Autodesk Inventor part; units mm, degrees
ref_plane "YZ Plane" through (0, 0, 0) normal (1, 0, 0) x (0, 1, 0)
ref_plane "XZ Plane" through (0, 0, 0) normal (0, 1, 0) x (-1, 0, 0)
ref_plane "XY Plane" through (0, 0, 0) normal (0, 0, 1) x (1, 0, 0)
sketch "Sketch1" plane through (0, 0, -12.5) normal (0, 1, 0) x (-1, 0, 0)
  line L0 (-27.5, 12.5) -> (27.5, 12.5)
  line L1 (27.5, 12.5) -> (27.5, 37.5)
  line L2 (27.5, 37.5) -> (15.5, 37.5)
  line L3 (15.5, 37.5) -> (18.5, 31.5)
  line L4 (18.5, 31.5) -> (-18.5, 31.5)
  line L5 (-18.5, 31.5) -> (-15.5, 37.5)
  line L6 (-15.5, 37.5) -> (-27.5, 37.5)
  line L7 (-27.5, 37.5) -> (-27.5, 12.5)
  line L8 (0, 7.5) -> (0, 42.5)
  line L9 (-38.5, 12.5) -> (38.5, 12.5)
  point P0 (0, 12.5)
  point P1 (0, 12.5)
  dimension "Base_Width" = 55
  dimension "Base_Height" = 25
  dimension "Slider_Shelf" = 12
  dimension "d3" = 9
  dimension "d2" = 6
extrude "Extrusion1" add sketch "Sketch1" along normal mid plane 120
sketch "Sketch4" plane through (-18.5, 60, 19) normal (0, 0, 1) x (1, 0, 0)
  line L0 (11, -110) -> (26, -110)
  line L1 (31, -105) -> (31, -15)
  line L2 (26, -10) -> (11, -10)
  line L3 (6, -15) -> (6, -105)
  arc A0 (6, -105) -> (11, -110) centre (11, -105) ccw
  arc A1 (26, -110) -> (31, -105) centre (26, -105) ccw
  arc A2 (31, -15) -> (26, -10) centre (26, -15) ccw
  arc A3 (11, -10) -> (6, -15) centre (11, -15) ccw
  line L4 (-20, -60) -> (57, -60)
  line L5 (18.5, 24) -> (18.5, -144)
  line L6 (-9, -120) -> (-9, 0)
  line L7 (37, 0) -> (0, 0)
  dimension "StopPlate_DP" = 5
  dimension "d25" = 100
  dimension "d26" = 25
extrude "Extrusion2" cut sketch "Sketch4" against normal through all
sketch "Sketch6" plane through (0, -60, -12.5) normal (0, -1, 0) x (1, 0, 0)
  line L0 (27.5, 37.5) -> (27.5, 12.5)
  line L1 (-27.5, 12.5) -> (27.5, 12.5)
  line L2 (27.5, 12.5) -> (27.5, 57)
  line L3 (27.5, 57) -> (-27.5, 57)
  line L4 (-27.5, 57) -> (-27.5, 12.5)
  point P0 (0, 12.5)
  dimension "EndBlock_HT" = 44.5
extrude "Extrusion4" add sketch "Sketch6" along normal blind 15
mirror "Mirror1" about plane through (0, 0, 0) normal (0, 1, 0) of "Extrusion4"
sketch "Sketch7" plane through (0, -75, -12.5) normal (0, -1, 0) x (1, 0, 0)
  line L0 (-27.5, 57) -> (27.5, 57)
  line L1 (0, 65.9) -> (0, 3.6)
  point P0 (0, 12.5)
  point P1 (0, 46.5)
  dimension "d39" = 10.5
hole "Hole1" at (0, -75, 34) direction (0, 1, 0) diameter 12 depth 75
sketch "Sketch14" plane through (0, -75, -12.5) normal (0, -1, 0) x (1, 0, 0)
  line L0 (27.5, 12.5) -> (-27.5, 12.5)
  line L1 (0, 65.9) -> (0, 3.6)
  point P0 (0, 12.5)
  point P1 (0, 20.5)
  dimension "d83" = 8
hole "Hole5" at (0, -75, 8) direction (0, 1, 0) diameter 6 depth 15 tip angle 118 countersink diameter 10.4 countersink angle 90
sketch "Sketch9" plane through (0, -60, -12.5) normal (0, -1, 0) x (1, 0, 0)
  circle A0 centre (0, 20.5) radius 5.2
  point P0 (0, 12.5)
hole "Hole3" at (0, -60, 8) direction (0, 1, 0) diameter 4.134 depth 8 tip angle 118
pattern_linear "Rectangular Pattern2" count 3 spacing 19.5 along (-1, 0, 0) of "Hole3", "Hole5" first direction both ways yes
mirror "Mirror2" about plane through (0, 0, 0) normal (0, 1, 0) of "Hole3", "Rectangular Pattern2", "Hole5"
sketch "Sketch11" plane through (-27.5, 60, 44.5) normal (0, -1, 0) x (1, 0, 0)
  line L0 (0, 0) -> (55, 0)
  line L1 (0, -44.5) -> (0, 0)
  line L2 (55, 0) -> (55, -44.5)
  point P0 (27.5, -44.5)
  point P1 (10, -9)
  point P2 (45, -9)
  dimension "d103" = 9
  dimension "d104" = 10
  dimension "d105" = 10
hole "Hole6" at (-17.5, 60, 35.5) at (17.5, 60, 35.5) direction (0, 1, 0) diameter 4.134 depth 10 tip angle 118
thread "Thread1"
chamfer "Chamfer1" distance 3 angle 45 6 edges at (-27.5, -67.5, 44.5) (27.5, -67.5, 44.5) (27.5, 67.5, 44.5) (-27.5, 67.5, 44.5) (27.5, 0, 25) (-27.5, 0, 25)
equation "\"d89\" = EndBlock_DP"
properties part number "Base"
The listing builds one solid part. Answer for the finished solid, in the listing's coordinates (mm). A direction names the side the tool comes from. Round coordinates to 2 decimals unless told otherwise and drop trailing zeros. Order: outer loops, then holes, each group sorted by start corner. A loop starts at its lowest first (then second) coordinate and runs counter-clockwise, first axis right, second up. Notation, with made-up numbers: (10, 42) -> (41, 42) arc R23 ccw to (41, 57) -> close; hole circle Ø1 at (5.5, -10.5). An arc over 180 degrees is marked (long way). Answer as CSV lines item,"result". Start each with the question number.
(1) For a pull along Y with two mould halves and no side action, classify faces 5 (the face through (0, -75, 23)), 6 (the face through (26, -0.8, 23.5)), 7 (the face through (16.838, 66.31, 6.616)) as +Y half, -Y half, draft (parallel to the pull), parting line (faces both ways), or undercut.
(2) Flat-ended cylindrical pins translate along their axes: pin 1 Ø3.5 at (x, z) = (0, 8) entering from +Y; pin 2 Ø6 at (x, y) = (15.5, -55.5) entering from +Z; pin 3 Ø2.5 at (x, z) = (19.5, 8) entering from -Y. Find the tip coordinate at first contact, or state that the pin passes through.
(3) The part is cut by section A-A (y = 4). Determine the outline of the cut face in (x, z).
(4) A tool of negligible diameter and unlimited length cuts with its end or side. For faces 1 (the face through (0, 67, 44.5)), 2 (the face through (12.5, -1, 10)), 3 (the face through (17.45, -55.67, 8.27)), 4 (the face through (-17, -1, 22)), from which of +Z, -Z, +X, -X, +Y, -Y can it reach the whole face along a straight path? Write none if from no direction.
(5) Find the intervals of material crossed by probe 1 along X at (y, z) = (54, 8); probe 2 along X at (y, z) = (64, 35.5); probe 3 along X at (y, z) = (-67, 8), in increasing order. Write a range as from..to.
Evaluation:
1,face 5,"-Y half"
1,face 6,"undercut"
1,face 7,"draft"
2,pin 1,"y = 51.81"
2,pin 2,"z = 25"
2,pin 3,"y = -51.51"
3,outline,"(-27.5, 0) -> (-12.5, 0) -> (-12.5, 19) -> (-18.5, 19) -> (-15.5, 25) -> (-24.5, 25) -> (-27.5, 22) -> close; (12.5, 0) -> (27.5, 0) -> (27.5, 22) -> (24.5, 25) -> (15.5, 25) -> (18.5, 19) -> (12.5, 19) -> close"
4,face 1,"+Z, +X, -X, +Y, -Y"
4,face 2,"+Z, -Z"
4,face 3,"-Y"
4,face 4,"none"
5,probe 1,"-27.5..-21.57, -17.43..-2.07, 2.07..17.43, 21.57..27.5"
5,probe 2,"-27.5..-19.57, -15.43..15.43, 19.57..27.5"
5,probe 3,"-27.5..-22.5, -16.5..-3, 3..16.5, 22.5..27.5"
